CAD build for the part. Positions are in the model's coordinates, mm. Give positions to 0.01 mm unless a question says otherwise; leave off trailing zeros.
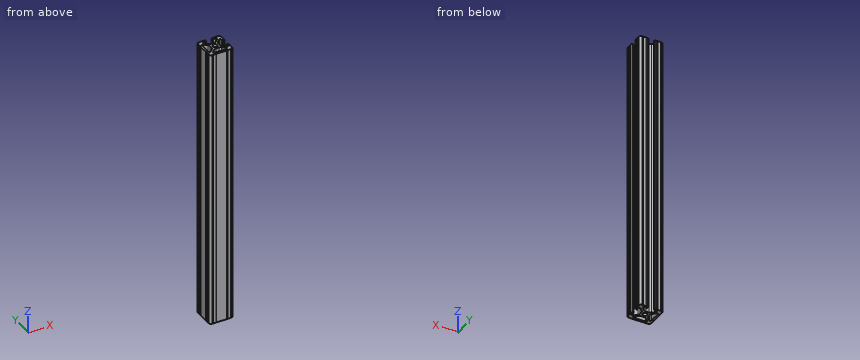
Autodesk Inventor part; units mm, degrees
ref_plane "YZ Plane" through (0, 0, 0) normal (1, 0, 0) x (0, 1, 0)
ref_plane "XZ Plane" through (0, 0, 0) normal (0, 1, 0) x (-1, 0, 0)
ref_plane "XY Plane" through (0, 0, 0) normal (0, 0, 1) x (1, 0, 0)
sketch "Sketch1" plane through (0, 0, 0) normal (0, 0, 1) x (1, 0, 0)
  circle A0 centre (0, 0) radius 2.6035
  arc A1 (-8.737, 7.1292) -> (-10.4902, 6.4021) centre (-9.4628, 6.4021) ccw
  line L0 (-5.4405, 3.8388) -> (-8.737, 7.1292)
  arc A2 (-4.5085, 1.5917) -> (-5.4405, 3.8388) centre (-7.6835, 1.5917) ccw
  line L1 (-4.5085, -1.5917) -> (-4.5085, 1.5917)
  arc A3 (-5.4405, -3.8388) -> (-4.5085, -1.5917) centre (-7.6835, -1.5917) ccw
  line L2 (-8.7534, -7.1457) -> (-5.4405, -3.8388)
  arc A4 (-10.4902, -6.4254) -> (-8.7534, -7.1457) centre (-9.4724, -6.4254) ccw
  line L3 (-10.4902, 6.4021) -> (-10.4902, -6.4254)
  arc A5 (-7.1537, -8.6712) -> (-6.436, -10.4062) centre (-6.436, -9.3902) ccw
  line L4 (-3.9003, -5.4237) -> (-7.1537, -8.6712)
  arc A6 (-1.6573, -4.4958) -> (-3.9003, -5.4237) centre (-1.6573, -7.6708) ccw
  line L5 (1.6573, -4.4958) -> (-1.6573, -4.4958)
  arc A7 (3.9003, -5.4237) -> (1.6573, -4.4958) centre (1.6573, -7.6708) ccw
  line L6 (7.1478, -8.6653) -> (3.9003, -5.4237)
  arc A8 (6.4276, -10.4062) -> (7.1478, -8.6653) centre (6.4276, -9.3868) ccw
  line L7 (-6.436, -10.4062) -> (6.4276, -10.4062)
  arc A9 (6.3331, -12.7) -> (5.3171, -12.7) centre (5.8251, -12.7) ccw
  line L8 (6.3331, -12.7) -> (9.5504, -12.7)
  arc A10 (10.5664, -12.6998) -> (9.5504, -12.7) centre (10.0584, -12.7) ccw
  arc A11 (10.5664, -12.6998) -> (12.6998, -10.5664) centre (10.5918, -10.5918) ccw
  arc A12 (12.7, -9.5504) -> (12.6998, -10.5664) centre (12.7, -10.0584) ccw
  line L9 (12.7, -9.5504) -> (12.7, -6.3331)
  arc A13 (12.7, -5.3171) -> (12.7, -6.3331) centre (12.7, -5.8251) ccw
  line L10 (12.7, -5.3171) -> (12.7, -4.2875)
  arc A14 (12.7, -4.2875) -> (11.651, -3.2385) centre (11.651, -4.2875) ccw
  line L11 (11.651, -3.2385) -> (11.5392, -3.2385)
  arc A15 (11.5392, -3.2385) -> (10.4902, -4.2875) centre (11.5392, -4.2875) ccw
  line L12 (10.4902, -4.2875) -> (10.4902, -6.4021)
  arc A16 (8.737, -7.1292) -> (10.4902, -6.4021) centre (9.4628, -6.4021) ccw
  line L13 (8.737, -7.1292) -> (5.4405, -3.8388)
  arc A17 (4.5085, -1.5917) -> (5.4405, -3.8388) centre (7.6835, -1.5917) ccw
  line L14 (4.5085, -1.5917) -> (4.5085, 1.5917)
  arc A18 (5.4405, 3.8388) -> (4.5085, 1.5917) centre (7.6835, 1.5917) ccw
  line L15 (5.4405, 3.8388) -> (8.737, 7.1292)
  arc A19 (10.4902, 6.4021) -> (8.737, 7.1292) centre (9.4628, 6.4021) ccw
  line L16 (10.4902, 6.4021) -> (10.4902, 4.2875)
  arc A20 (10.4902, 4.2875) -> (11.5392, 3.2385) centre (11.5392, 4.2875) ccw
  line L17 (11.5392, 3.2385) -> (11.651, 3.2385)
  arc A21 (11.651, 3.2385) -> (12.7, 4.2875) centre (11.651, 4.2875) ccw
  line L18 (12.7, 4.2875) -> (12.7, 5.3171)
  arc A22 (12.7, 6.3331) -> (12.7, 5.3171) centre (12.7, 5.8251) ccw
  line L19 (12.7, 6.3331) -> (12.7, 9.5504)
  arc A23 (12.6998, 10.5664) -> (12.7, 9.5504) centre (12.7, 10.0584) ccw
  arc A24 (12.6998, 10.5664) -> (10.5664, 12.6998) centre (10.5918, 10.5918) ccw
  arc A25 (9.5504, 12.7) -> (10.5664, 12.6998) centre (10.0584, 12.7) ccw
  line L20 (9.5504, 12.7) -> (6.3331, 12.7)
  arc A26 (5.3171, 12.7) -> (6.3331, 12.7) centre (5.8251, 12.7) ccw
  line L21 (5.3171, 12.7) -> (4.2875, 12.7)
  arc A27 (4.2875, 12.7) -> (3.2385, 11.651) centre (4.2875, 11.651) ccw
  line L22 (3.2385, 11.651) -> (3.2385, 11.5392)
  arc A28 (3.2385, 11.5392) -> (4.2875, 10.4902) centre (4.2875, 11.5392) ccw
  line L23 (4.2875, 10.4902) -> (6.4768, 10.4902)
  arc A29 (7.2072, 8.7246) -> (6.4768, 10.4902) centre (6.4768, 9.4563) ccw
  line L24 (7.2072, 8.7246) -> (3.9003, 5.4237)
  arc A30 (1.6573, 4.4958) -> (3.9003, 5.4237) centre (1.6573, 7.6708) ccw
  line L25 (1.6573, 4.4958) -> (-1.5537, 4.4958)
  arc A31 (-3.7967, 5.4237) -> (-1.5537, 4.4958) centre (-1.5537, 7.6708) ccw
  line L26 (-3.7967, 5.4237) -> (-7.1342, 8.7551)
  arc A32 (-6.4164, 10.4902) -> (-7.1342, 8.7551) centre (-6.4164, 9.4742) ccw
  line L27 (-6.4164, 10.4902) -> (-4.2875, 10.4902)
  arc A33 (-4.2875, 10.4902) -> (-3.2385, 11.5392) centre (-4.2875, 11.5392) ccw
  line L28 (-3.2385, 11.5392) -> (-3.2385, 11.651)
  arc A34 (-3.2385, 11.651) -> (-4.2875, 12.7) centre (-4.2875, 11.651) ccw
  line L29 (-4.2875, 12.7) -> (-5.3171, 12.7)
  arc A35 (-6.3331, 12.7) -> (-5.3171, 12.7) centre (-5.8251, 12.7) ccw
  line L30 (-6.3331, 12.7) -> (-9.5504, 12.7)
  arc A36 (-10.5664, 12.6998) -> (-9.5504, 12.7) centre (-10.0584, 12.7) ccw
  arc A37 (-10.5664, 12.6998) -> (-12.6998, 10.5664) centre (-10.5918, 10.5918) ccw
  arc A38 (-12.7, 9.5504) -> (-12.6998, 10.5664) centre (-12.7, 10.0584) ccw
  line L31 (-12.7, 9.5504) -> (-12.7, 6.3331)
  arc A39 (-12.7, 5.3171) -> (-12.7, 6.3331) centre (-12.7, 5.8251) ccw
  line L32 (-12.7, 5.3171) -> (-12.7, -5.3171)
  arc A40 (-12.7, -6.3331) -> (-12.7, -5.3171) centre (-12.7, -5.8251) ccw
  line L33 (-12.7, -6.3331) -> (-12.7, -9.5504)
  arc A41 (-12.6998, -10.5664) -> (-12.7, -9.5504) centre (-12.7, -10.0584) ccw
  arc A42 (-12.6998, -10.5664) -> (-10.5664, -12.6998) centre (-10.5918, -10.5918) ccw
  arc A43 (-9.5504, -12.7) -> (-10.5664, -12.6998) centre (-10.0584, -12.7) ccw
  line L34 (-9.5504, -12.7) -> (-6.3331, -12.7)
  arc A44 (-5.3171, -12.7) -> (-6.3331, -12.7) centre (-5.8251, -12.7) ccw
  line L35 (-5.3171, -12.7) -> (5.3171, -12.7)
extrude "Extrusion1" add sketch "Sketch1" against normal blind 304.8
properties part number "1002"
1. Drop flat-ended pins along their axis: pin 1 (1.6 mm diameter, centred on y = 0.5, z = -172, fed in from +X); pin 2 (1.6 mm diameter, centred on x = 0, z = -166.5, fed in from +Y). Give the stop position or say it passes through.
Responses:
pin 1: stops at x = 4.51
pin 2: stops at y = 4.5
2. Saw through at A-A, the plane z = -214. Count the separate pieces of the cut face and the enclosed holes in it, and give its area (3 significant figures).
Responses:
separate pieces: 1
enclosed holes: 3
area: 313 mm2
3. Probe line 1 along Y through (x, z) = (0, -108.5); line 2 along Y through (x, z) = (-9.25, -263); line 3 along Y through (x, z) = (2.25, -36). List the from-to ranges inside material, lowest first.
Responses:
line 1: y = -12.7 to -10.41, -4.5 to -2.6, 2.6 to 4.5
line 2: y = -12.7 to -7.42, 7.41 to 12.7
line 3: y = -12.7 to -10.41, -4.55 to -1.31, 1.31 to 4.55
